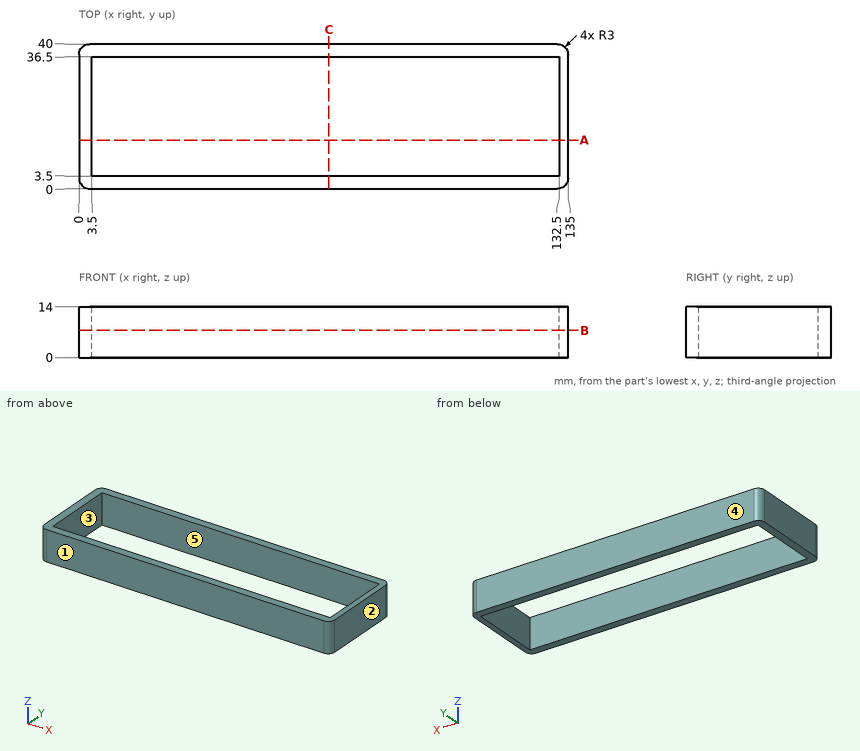
The drawing under review shows one solid part. Ordinate dimensions are in mm from its lowest x, y, z. A direction names the side the tool comes from. Coordinates: 2 decimals unless noted, no trailing zeros. Write each loop counter-clockwise with the first axis right and the second up, starting at its lowest first coordinate (ties: lowest second). Pieces come first, ordered by that corner, then holes.
1) Add section C-C (x = 69). Write out the cut boundary in (y, z), plus the area to 3 significant figures.
2) Add section A-A (y = 13.5). Write out the cut boundary in (x, z).
3) To check wall thickness, follow L1, parallel to X at y = 8.5, z = 7.75; L2, parallel to Y at x = 33.5, z = 3.75. State the ranges of each line that lie inside material, in increasing order.
4) Machinability: for the marked faces 4 and 5, which of the approach directions +Z, -Z, +X, -X, +Y, -Y give a long, thin tool a straight path to every point of the face, cutting with its end or side? Answer none if there is none.
5) Add section B-B (z = 7.5). Write out the cut boundary in (x, y).
6) Mouldability with a two-part tool opening along Y and no side actions: class the marked faces 1, 2 and 3 as +Y half, -Y half, draft (parallel to the pull), parting line (faces both ways), or undercut.
Check result:
1. outline: (0, 0) - (3.5, 0) - (3.5, 14) - (0, 14) - close; (36.5, 0) - (40, 0) - (40, 14) - (36.5, 14) - close
1. area: 98.0 mm2
2. outline: (0, 0) - (3.5, 0) - (3.5, 14) - (0, 14) - close; (132.5, 0) - (135, 0) - (135, 14) - (132.5, 14) - close
3. L1: x = 0 to 3.5, 132.5 to 135
3. L2: y = 0 to 3.5, 36.5 to 40
4. face 4: +Z, -Z, +X, -X, +Y
4. face 5: +Z, -Z
5. outline: (0, 3) arc R3 ccw to (3, 0) - (132, 0) arc R3 ccw to (135, 3) - (135, 37) arc R3 ccw to (132, 40) - (3, 40) arc R3 ccw to (0, 37) - close; hole (3.5, 3.5) - (132.5, 3.5) - (132.5, 36.5) - (3.5, 36.5) - close
6. face 1: -Y half
6. face 2: draft
6. face 3: undercut
